Can you work these out from the model? Positions are in its coordinate system, mm. Face numbers are marked on the shaded views. A direction names the side the tool comes from. Give positions to 0.01 mm unless a question says otherwise; leave off trailing zeros. Loops run counter-clockwise (first coordinate to the right, second up) from the corner with the lowest first, then second, coordinate; pieces in that order, holes last.
from build123d import *

# Parameters (mm, degrees)
F1_DEPTH = 72
F3_DEPTH = 4
F5_DEPTH = 4
F7_DEPTH = 25
F8_R     = 3
F9_DEPTH = 5.5


with BuildPart() as f1:
    # F0 (on Top) → F1 (new body)
    with BuildSketch(Plane.XY):
        Polygon((-232, 28.7712871801), (-232, 9), (-232, -7), (7, -7), (7, 102), (-170.6706311353, 102), align=None)
        Polygon((0, 9), (0, 0), (-11.2000130415, 0), (-29.7000130415, 0), (-48.2000130415, 0), (-66.7000130415, 0), (-85.2000130415, 0), (-103.7000130415, 0), (-122.2000130415, 0), (-140.7000130415, 0), (-159.2000130415, 0), (-177.7000130415, 0), (-196.2000130415, 0), (-214.7000130415, 0), (-225, 0), (-225, 9), (-225, 19.009443), (-216.0657793283, 19.009443), (-216.0657793283, 33.8660545808), (-218.6024326595, 33.8660545808), (-176.2169181556, 84.4753585209), (-160.9487113722, 84.4753585209), (-160.9487113722, 95), (0, 95), (0, 80.24520114), (-12.4263259421, 80.2028560212), (-12.3839236644, 67.7597565904), (0, 67.7597565904), (0, 30.28925322), (-9.0186540037, 30.28925322), (-9.0186540037, 19.0464295447), (0, 19.0464295447), align=None, mode=Mode.SUBTRACT)
    extrude(amount=F1_DEPTH)

    # F2 (on Top) → F3 (join)
    with BuildSketch(Plane.XY):
        Polygon((-170.6706311353, 102), (-232, 28.7712871801), (-232, -7), (7, -7), (7, 102), align=None)
    extrude(amount=-F3_DEPTH)

    # F4 (on face) → F5 (join)
    with BuildSketch(Plane.XY.offset(72)):
        Polygon((7, 102), (-170.6706311353, 102), (-232, 28.7712871801), (-232, -7), (7, -7), align=None)
        Polygon((-230, -5), (-230, 28.0444074988), (-169.7368749983, 100), (5, 100), (5, -5), align=None, mode=Mode.SUBTRACT)
    extrude(amount=F5_DEPTH)

    # F6 (on face) → F7 (cut)
    with BuildSketch(Plane.YZ.offset(7)):
        with BuildLine():
            Line((4.5232147723, 36), (14.5232147723, 36))
            ThreePointArc((14.5232147723, 36), (9.5232147723, 41), (4.5232147723, 36))
        make_face()
        with BuildLine():
            ThreePointArc((4.5232147723, 36), (9.5232147723, 31), (14.5232147723, 36))
            Line((14.5232147723, 36), (4.5232147723, 36))
        make_face()
    extrude(amount=-F7_DEPTH, mode=Mode.SUBTRACT)

    # F8 (on face) → F9 (cut)
    with BuildSketch(Plane.XY.offset(72)):
        with Locations((-167.3095971346, 89.7376792604)):
            Circle(F8_R)
        with Locations((-222.2577780485, 26.4377487904)):
            Circle(F8_R)
        with Locations((-5.7860915549, 73.9813063058)):
            Circle(F8_R)
        with Locations((-3.1610322185, 24.6678413823)):
            Circle(F8_R)
    extrude(amount=-F9_DEPTH, mode=Mode.SUBTRACT)


solid = f1.part
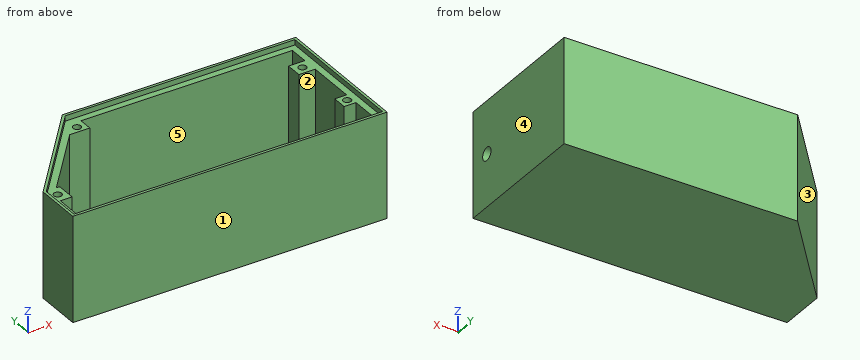
(1) Suppose I cut it at B-B on z = 25. List the corners of the cut face in (x, y) for me, plus the area to 3 significant figures.
Returned:
outline: (-232, -7) - (7, -7) - (7, 102) - (-170.67, 102) - (-232, 28.77) - close; hole (-225, 0) - (0, 0) - (0, 19.05) - (-9.02, 19.05) - (-9.02, 30.29) - (0, 30.29) - (0, 67.76) - (-12.38, 67.76) - (-12.43, 80.2) - (0, 80.25) - (0, 95) - (-160.95, 95) - (-160.95, 84.48) - (-176.22, 84.48) - (-218.6, 33.87) - (-216.07, 33.87) - (-216.07, 19.01) - (-225, 19.01) - close
area: 4,890 mm2
(2) Will these pins go through, and if not, where does the flat tip stop? P1, Ø1.2, axis at y = 31.5, z = 73, coming from the -X side; P2, Ø5, axis at y = 37, z = 8, coming from the -X side; P3, Ø7, axis at x = -5.79, y = 73.98, coming from the +Z side.
Returned:
P1: stops at x = -230.22
P2: stops at x = -227.2
P3: stops at z = 72
(3) Suppose I cut it at A-A on x = -100. List the corners of the cut face in (y, z) for me, plus the area to 3 significant figures.
Returned:
outline: (-7, -4) - (102, -4) - (102, 76) - (100, 76) - (100, 72) - (95, 72) - (95, 0) - (0, 0) - (0, 72) - (-5, 72) - (-5, 76) - (-7, 76) - close
area: 1,460 mm2
(4) Suppose I cut it at D-D on y = 44.5. List the corners of the cut face in (x, z) for me, plus the area to 3 significant figures.
Returned:
outline: (-218.83, -4) - (7, -4) - (7, 76) - (5, 76) - (5, 72) - (0, 72) - (0, 0) - (-209.7, 0) - (-209.7, 72) - (-216.22, 72) - (-216.22, 76) - (-218.83, 76) - close
area: 2,080 mm2
(5) Please list where these lines run through material, in increasing order: probe 1 along Y at (x, z) = (2, 36); probe 2 along Y at (x, z) = (-101.5, 20); probe 3 along X at (y, z) = (4.5, 68).
Returned:
probe 1: y = -7 to 4.52, 14.52 to 102
probe 2: y = -7 to 0, 95 to 102
probe 3: x = -232 to -225, 0 to 7
(6) Thinking about a two-plate mould opening in Y: for the marked faces 1, 2 and 3, which applies, pulls with the +Y half, pulls with the -Y half, needs draft (parallel to the pull), parting line crosses it, or undercut?
Returned:
face 1: pulls with the -Y half
face 2: undercut
face 3: pulls with the +Y half
(7) Which directions (+Z, -Z, +X, -X, +Y, -Y) give clear straight access to the entire face, cutting with the end or side of a thin tool? Please do the marked faces 4 and 5.
Returned:
face 4: +Z, -Z, +X, +Y, -Y
face 5: +Z
(8) Suppose I cut it at C-C on z = 36. List the corners of the cut face in (x, y) for me, plus the area to 3 significant figures.
Returned:
outline: (-232, -7) - (7, -7) - (7, 4.52) - (0, 4.52) - (0, 0) - (-225, 0) - (-225, 19.01) - (-216.07, 19.01) - (-216.07, 33.87) - (-218.6, 33.87) - (-176.22, 84.48) - (-160.95, 84.48) - (-160.95, 95) - (0, 95) - (0, 80.25) - (-12.43, 80.2) - (-12.38, 67.76) - (0, 67.76) - (0, 30.29) - (-9.02, 30.29) - (-9.02, 19.05) - (0, 19.05) - (0, 14.52) - (7, 14.52) - (7, 102) - (-170.67, 102) - (-232, 28.77) - close
area: 4,820 mm2
